```python
from build123d import *

# Parameters (mm, degrees)
BOSS_EXTRUDE1_DEPTH = 5
BOSS_EXTRUDE2_DEPTH = 10


with BuildPart() as part:
    # Sketch1 → Boss-Extrude1 (new, symmetric)
    with BuildSketch(Plane.XY):
        Polygon((51.5, 0), (0, 0), (0, -50), (15, -50), (15, -15), (51.5, -15), align=None)
    extrude(amount=BOSS_EXTRUDE1_DEPTH, both=True)

    # Sketch2 → Boss-Extrude2 (add)
    with BuildSketch(Plane.XZ.offset(50)):
        Polygon((22.832157544, -5), (18, -6.284621916), (15, 5), (18, 16.284621916), (22.832157544, 15), (20.173672375, 5), align=None)
        Polygon((15, -5), (17.658485169, -5), (15, 5), align=None)
        Polygon((18, 16.284621916), (15, 5), (20.173672375, 5), (22.832157544, 15), align=None)
    extrude(amount=-BOSS_EXTRUDE2_DEPTH)


solid = part.part
```
Check sheet for the modelled part. Datum: model origin and axes. Units: mm. A direction names the side the tool comes from. Give positions to 0.01 mm unless a question says otherwise; leave off trailing zeros. Write each loop counter-clockwise with the first axis right and the second up, starting at its lowest first coordinate (ties: lowest second). Pieces come first, ordered by that corner, then holes. Notation, with made-up numbers: (-1, 16) -> (7, 16) arc R17 ccw to (7, 49) -> close; hole circle Ø6 at (44.25, 82). An arc over 180 degrees is marked (long way). Use CSV: the item, a comma, the result in double quotes. Start each with the question number.
Q1. Scan lines: line 1 along Y through (x, z) = (29.5, 0.5); line 2 along X through (y, z) = (-18.5, -2.5); line 3 along Y through (x, z) = (15.5, -0.5). Record each from-to range of solid material in increasing order.
Q2. Depth check by flat-ended pin: P1, Ø5, axis at y = -33, z = 0.5, coming from the +X side; P2, Ø25, axis at x = 35.5, y = -14.5, coming from the -Z side; P3, Ø4, axis at x = 41.5, z = 1.5, coming from the -Y side; P4, Ø1, axis at x = 40.5, z = 6.5, coming from the +Y side. Enter the tip coordinate at first touch or a pass-through.
Q3. Cross-section at B-B on z = -1.5. Enter the section's corners in (x, y), and give its area (3 significant figures).
Q4. Cross-section at C-C on x = 12. Enter the section's corners in (y, z), and give its area (3 significant figures).
Q5. Cross-section at A-A on y = -43.5. Enter the section's corners in (x, z).
Q6. Tool access check on faces 1 (the flat face through (21.52, -45.07, 10.07)), 2 (the flat face through (21.484, -45.07, 0.07)), 3 (the flat face through (33, -15, 0)). Record the directions out of +Z, -Z, +X, -X, +Y, -Y that give a thin tool (end or side, any length) a straight path to the whole face; none if there is none.
Q7. Cross-section at D-D on y = -7. Enter the section's corners in (x, z), and give its area (3 significant figures).
Working result:
1,line 1,"y = -15 to 0"
1,line 2,"x = 0 to 15"
1,line 3,"y = -50 to -40, -15 to 0"
2,P1,"stops at x = 15"
2,P2,"stops at z = -5"
2,P3,"stops at y = -15"
2,P4,"passes through"
3,outline,"(0, -50) -> (21.9, -50) -> (21.9, -40) -> (15, -40) -> (15, -15) -> (51.5, -15) -> (51.5, 0) -> (0, 0) -> close"
3,area,"1,370 mm^2"
4,outline,"(-50, -5) -> (0, -5) -> (0, 5) -> (-50, 5) -> close"
4,area,"500 mm^2"
5,outline,"(0, -5) -> (17.66, -5) -> (18, -6.28) -> (22.83, -5) -> (20.17, 5) -> (22.83, 15) -> (18, 16.28) -> (15, 5) -> (0, 5) -> close"
6,face 1,"+X, +Y, -Y"
6,face 2,"+X, -Y"
6,face 3,"+Z, -Z, +X"
7,outline,"(0, -5) -> (51.5, -5) -> (51.5, 5) -> (0, 5) -> close"
7,area,"515 mm^2"
